from build123d import *

# Parameters (mm, degrees)
AUFSATZ_LINEAR_AUSTRAGEN1_DEPTH = 3
AUFSATZ_LINEAR_AUSTRAGEN2_DEPTH = 83.5
SKIZZE5_R                       = 1.05
SCHNITT_LINEAR_AUSTRAGEN2_DEPTH = 13


with BuildPart() as part:
    # Skizze2 → Aufsatz-Linear austragen1 (new body)
    with BuildSketch(Plane.XY):
        with BuildLine():
            ThreePointArc((18.5, 0), (13.081475452, 13.081475452), (0, 18.5))
            Line((0, 18.5), (0, 17.2))
            ThreePointArc((0, 17.2), (0.777817459, 16.877817459), (1.1, 16.1))
            ThreePointArc((1.1, 16.1), (1.099839478, 16.081208438), (1.099357959, 16.06242236))
            ThreePointArc((1.099357959, 16.06242236), (0.764416312, 15.309008406), (0, 15))
            Line((0, 15), (0, 14.3))
            ThreePointArc((0, 14.3), (0.777817459, 13.977817459), (1.1, 13.2))
            ThreePointArc((1.1, 13.2), (1.099761155, 13.177078356), (1.099044724, 13.154166667))
            ThreePointArc((1.099044724, 13.154166667), (0.761440521, 12.40614338), (0, 12.1))
            Line((0, 12.1), (0, 11.25))
            ThreePointArc((0, 11.25), (0.777817459, 10.927817459), (1.1, 10.15))
            ThreePointArc((1.1, 10.15), (1.099595894, 10.120186092), (1.098383874, 10.090394089))
            ThreePointArc((1.098383874, 10.090394089), (0.756450097, 9.35138667), (0, 9.05))
            Line((0, 9.05), (0, 8.35))
            ThreePointArc((0, 8.35), (0.777817459, 8.027817459), (1.1, 7.25))
            ThreePointArc((1.1, 7.25), (1.099207253, 7.208245771), (1.096830153, 7.166551724))
            ThreePointArc((1.096830153, 7.166551724), (0.747732204, 6.443218399), (0, 6.15))
            Line((0, 6.15), (0, 0))
            Line((0, 0), (6.15, 0))
            ThreePointArc((6.15, 0), (6.443218399, 0.747732204), (7.166551724, 1.096830153))
            ThreePointArc((7.166551724, 1.096830153), (7.997732204, 0.806781601), (8.35, 0))
            Line((8.35, 0), (9.05, 0))
            ThreePointArc((9.05, 0), (9.35138667, 0.756450097), (10.090394089, 1.098383874))
            ThreePointArc((10.090394089, 1.098383874), (10.906450097, 0.79861333), (11.25, 0))
            Line((11.25, 0), (12.1, 0))
            ThreePointArc((12.1, 0), (12.40614338, 0.761440521), (13.154166667, 1.099044724))
            ThreePointArc((13.154166667, 1.099044724), (13.961440521, 0.79385662), (14.3, 0))
            Line((14.3, 0), (15, 0))
            ThreePointArc((15, 0), (15.309008406, 0.764416312), (16.06242236, 1.099357959))
            ThreePointArc((16.06242236, 1.099357959), (16.864416312, 0.790991594), (17.2, 0))
            Line((17.2, 0), (18.5, 0))
        make_face()
        with BuildLine():
            ThreePointArc((0, -18.5), (13.081475452, -13.081475452), (18.5, 0))
            Line((18.5, 0), (17.2, 0))
            ThreePointArc((17.2, 0), (16.864416312, -0.790991594), (16.06242236, -1.099357959))
            ThreePointArc((16.06242236, -1.099357959), (15.309008406, -0.764416312), (15, 0))
            Line((15, 0), (14.3, 0))
            ThreePointArc((14.3, 0), (13.961440521, -0.79385662), (13.154166667, -1.099044724))
            ThreePointArc((13.154166667, -1.099044724), (12.40614338, -0.761440521), (12.1, 0))
            Line((12.1, 0), (11.25, 0))
            ThreePointArc((11.25, 0), (10.906450097, -0.79861333), (10.090394089, -1.098383874))
            ThreePointArc((10.090394089, -1.098383874), (9.35138667, -0.756450097), (9.05, 0))
            Line((9.05, 0), (8.35, 0))
            ThreePointArc((8.35, 0), (7.997732204, -0.806781601), (7.166551724, -1.096830153))
            ThreePointArc((7.166551724, -1.096830153), (6.443218399, -0.747732204), (6.15, 0))
            Line((6.15, 0), (0, 0))
            Line((0, 0), (0, -6.15))
            ThreePointArc((0, -6.15), (0.747732204, -6.443218399), (1.096830153, -7.166551724))
            ThreePointArc((1.096830153, -7.166551724), (1.099207253, -7.208245771), (1.1, -7.25))
            ThreePointArc((1.1, -7.25), (0.777817459, -8.027817459), (0, -8.35))
            Line((0, -8.35), (0, -9.05))
            ThreePointArc((0, -9.05), (0.756450097, -9.35138667), (1.098383874, -10.090394089))
            ThreePointArc((1.098383874, -10.090394089), (1.099595894, -10.120186092), (1.1, -10.15))
            ThreePointArc((1.1, -10.15), (0.777817459, -10.927817459), (0, -11.25))
            Line((0, -11.25), (0, -12.1))
            ThreePointArc((0, -12.1), (0.761440521, -12.40614338), (1.099044724, -13.154166667))
            ThreePointArc((1.099044724, -13.154166667), (1.099761155, -13.177078356), (1.1, -13.2))
            ThreePointArc((1.1, -13.2), (0.777817459, -13.977817459), (0, -14.3))
            Line((0, -14.3), (0, -15))
            ThreePointArc((0, -15), (0.764416312, -15.309008406), (1.099357959, -16.06242236))
            ThreePointArc((1.099357959, -16.06242236), (1.099839478, -16.081208438), (1.1, -16.1))
            ThreePointArc((1.1, -16.1), (0.777817459, -16.877817459), (0, -17.2))
            Line((0, -17.2), (0, -18.5))
        make_face()
        with BuildLine():
            Line((-17.2, 0), (-18.5, 0))
            ThreePointArc((-18.5, 0), (-13.081475452, -13.081475452), (0, -18.5))
            Line((0, -18.5), (0, -17.2))
            ThreePointArc((0, -17.2), (-0.790991594, -16.864416312), (-1.099357959, -16.06242236))
            ThreePointArc((-1.099357959, -16.06242236), (-0.764416312, -15.309008406), (0, -15))
            Line((0, -15), (0, -14.3))
            ThreePointArc((0, -14.3), (-0.79385662, -13.961440521), (-1.099044724, -13.154166667))
            ThreePointArc((-1.099044724, -13.154166667), (-0.761440521, -12.40614338), (0, -12.1))
            Line((0, -12.1), (0, -11.25))
            ThreePointArc((0, -11.25), (-0.79861333, -10.906450097), (-1.098383874, -10.090394089))
            ThreePointArc((-1.098383874, -10.090394089), (-0.756450097, -9.35138667), (0, -9.05))
            Line((0, -9.05), (0, -8.35))
            ThreePointArc((0, -8.35), (-0.806781601, -7.997732204), (-1.096830153, -7.166551724))
            ThreePointArc((-1.096830153, -7.166551724), (-0.747732204, -6.443218399), (0, -6.15))
            Line((0, -6.15), (0, 0))
            Line((0, 0), (-6.15, 0))
            ThreePointArc((-6.15, 0), (-6.443218399, -0.747732204), (-7.166551724, -1.096830153))
            ThreePointArc((-7.166551724, -1.096830153), (-7.997732204, -0.806781601), (-8.35, 0))
            Line((-8.35, 0), (-9.05, 0))
            ThreePointArc((-9.05, 0), (-9.35138667, -0.756450097), (-10.090394089, -1.098383874))
            ThreePointArc((-10.090394089, -1.098383874), (-10.906450097, -0.79861333), (-11.25, 0))
            Line((-11.25, 0), (-12.1, 0))
            ThreePointArc((-12.1, 0), (-12.40614338, -0.761440521), (-13.154166667, -1.099044724))
            ThreePointArc((-13.154166667, -1.099044724), (-13.961440521, -0.79385662), (-14.3, 0))
            Line((-14.3, 0), (-15, 0))
            ThreePointArc((-15, 0), (-15.309008406, -0.764416312), (-16.06242236, -1.099357959))
            ThreePointArc((-16.06242236, -1.099357959), (-16.864416312, -0.790991594), (-17.2, 0))
        make_face()
        with BuildLine():
            Line((0, 17.2), (0, 18.5))
            ThreePointArc((0, 18.5), (-13.081475452, 13.081475452), (-18.5, 0))
            Line((-18.5, 0), (-17.2, 0))
            ThreePointArc((-17.2, 0), (-16.864416312, 0.790991594), (-16.06242236, 1.099357959))
            ThreePointArc((-16.06242236, 1.099357959), (-15.309008406, 0.764416312), (-15, 0))
            Line((-15, 0), (-14.3, 0))
            ThreePointArc((-14.3, 0), (-13.961440521, 0.79385662), (-13.154166667, 1.099044724))
            ThreePointArc((-13.154166667, 1.099044724), (-12.40614338, 0.761440521), (-12.1, 0))
            Line((-12.1, 0), (-11.25, 0))
            ThreePointArc((-11.25, 0), (-10.906450097, 0.79861333), (-10.090394089, 1.098383874))
            ThreePointArc((-10.090394089, 1.098383874), (-9.35138667, 0.756450097), (-9.05, 0))
            Line((-9.05, 0), (-8.35, 0))
            ThreePointArc((-8.35, 0), (-7.997732204, 0.806781601), (-7.166551724, 1.096830153))
            ThreePointArc((-7.166551724, 1.096830153), (-6.443218399, 0.747732204), (-6.15, 0))
            Line((-6.15, 0), (0, 0))
            Line((0, 0), (0, 6.15))
            ThreePointArc((0, 6.15), (-0.747732204, 6.443218399), (-1.096830153, 7.166551724))
            ThreePointArc((-1.096830153, 7.166551724), (-0.806781601, 7.997732204), (0, 8.35))
            Line((0, 8.35), (0, 9.05))
            ThreePointArc((0, 9.05), (-0.756450097, 9.35138667), (-1.098383874, 10.090394089))
            ThreePointArc((-1.098383874, 10.090394089), (-0.79861333, 10.906450097), (0, 11.25))
            Line((0, 11.25), (0, 12.1))
            ThreePointArc((0, 12.1), (-0.761440521, 12.40614338), (-1.099044724, 13.154166667))
            ThreePointArc((-1.099044724, 13.154166667), (-0.79385662, 13.961440521), (0, 14.3))
            Line((0, 14.3), (0, 15))
            ThreePointArc((0, 15), (-0.764416312, 15.309008406), (-1.099357959, 16.06242236))
            ThreePointArc((-1.099357959, 16.06242236), (-0.790991594, 16.864416312), (0, 17.2))
        make_face()
    extrude(amount=AUFSATZ_LINEAR_AUSTRAGEN1_DEPTH)

    # Skizze4 → Aufsatz-Linear austragen2 (add)
    with BuildSketch(Plane.XY.offset(3)):
        Polygon((2.828427125, 6.363961031), (10.960155108, 14.495689014), (14.495689014, 10.960155108), (6.363961031, 2.828427125), align=None)
        Polygon((6.363961031, -2.828427125), (14.495689014, -10.960155108), (10.960155108, -14.495689014), (2.828427125, -6.363961031), align=None)
        Polygon((-2.828427125, -6.363961031), (-10.960155108, -14.495689014), (-14.495689014, -10.960155108), (-6.363961031, -2.828427125), align=None)
        Polygon((-6.363961031, 2.828427125), (-14.495689014, 10.960155108), (-10.960155108, 14.495689014), (-2.828427125, 6.363961031), align=None)
    extrude(amount=AUFSATZ_LINEAR_AUSTRAGEN2_DEPTH)

    # Skizze5 → Schnitt-Linear austragen2 (cut)
    with BuildSketch(Plane.XY.offset(86.5)):
        with Locations((-8.66205807, -8.66205807)):
            Circle(SKIZZE5_R)
        with Locations((-8.66205807, 8.66205807)):
            Circle(SKIZZE5_R)
        with Locations((8.66205807, 8.66205807)):
            Circle(SKIZZE5_R)
        with Locations((8.66205807, -8.66205807)):
            Circle(SKIZZE5_R)
    extrude(amount=-SCHNITT_LINEAR_AUSTRAGEN2_DEPTH, mode=Mode.SUBTRACT)


solid = part.part
Geometry: final body of the model. Coordinates: model frame, mm. A direction names the side the tool comes from. Give positions to 0.01 mm unless a question says otherwise; leave off trailing zeros. Loops run counter-clockwise (first coordinate to the right, second up) from the corner with the lowest first, then second, coordinate; pieces in that order, holes last. Notation, with made-up numbers: M 15,62 L 65,62 A8 ccw 65,69 Z; hole C 27,80 d6. An arc over 180 degrees is marked long. Put each result on its own line as item: value. Start each with the question number.
1) Pull-direction query (Y, two-part tool) for faces 5 (the flat face through (-7, -9, 86.5)), 6 (the cylindrical face through (-8.89, 7.637, 80.091)), 7 (the flat face through (6.837, 10.373, 44.166)); classes: pulls with the +Y half, pulls with the -Y half, needs draft (parallel to the pull), parting line crosses it, or undercut.
2) Cut plane C-C (x = -5). Output: boundary loops of the cut face in (y, z), then the cut area to 3 significant figures.
3) Cut plane A-A (z = 57). Output: boundary loops of the cut face in (x, y).
4) Contact query for flat-ended pins moving along their axis: pin 1 (1.5 mm diameter, centred on x = -7.5, z = 10.5, fed in from -Y); pin 2 (6 mm diameter, centred on x = -3, z = 67.5, fed in from -Y); pin 3 (8 mm diameter, centred on x = -11.5, z = 50.5, fed in from -Y). Output: stop coordinate, or through.
5) Access query for faces 1 (the flat face through (10.487, 6.951, 44.166)), 2 (the flat face through (-10.487, -6.951, 44.166)), 3 (the flat face through (-6.951, 10.487, 44.166)), 4 (the flat face through (-9, -9, 73.5)). Directions: +Z, -Z, +X, -X, +Y, -Y. A direction counts if a zero-diameter tool reaches every point of the face in a straight line with its end or side. Return the directions, or none.
6) Cut plane B-B (z = 81.5). Output: boundary loops of the cut face in (x, y).
7) Ray query, line 1 along Z through (x, y) = (-16, 5); line 2 along X through (y, z) = (-7, 81.5). Return the intervals inside material, ascending.
Verdict:
1. face 5: needs draft
1. face 6: undercut
1. face 7: pulls with the +Y half
2. outline: M -17.81,0 L 17.81,0 L 17.81,3 L 8.54,3 L 8.54,86.5 L 4.19,86.5 L 4.19,3 L -4.19,3 L -4.19,86.5 L -8.54,86.5 L -8.54,3 L -17.81,3 Z
2. area: 832 mm2
3. outline: M -14.5,-10.96 L -10.96,-14.5 L -2.83,-6.36 L -6.36,-2.83 Z; M -14.5,10.96 L -6.36,2.83 L -2.83,6.36 L -10.96,14.5 Z; M 2.83,-6.36 L 10.96,-14.5 L 14.5,-10.96 L 6.36,-2.83 Z; M 2.83,6.36 L 6.36,2.83 L 14.5,10.96 L 10.96,14.5 Z
4. pin 1: y = -11.79
4. pin 2: y = -9.54
4. pin 3: y = -14.5
5. face 1: +Z, +X
5. face 2: +Z, -X
5. face 3: +Z, +Y
5. face 4: +Z
6. outline: M -14.5,-10.96 L -10.96,-14.5 L -2.83,-6.36 L -6.36,-2.83 Z; M -14.5,10.96 L -6.36,2.83 L -2.83,6.36 L -10.96,14.5 Z; M 2.83,-6.36 L 10.96,-14.5 L 14.5,-10.96 L 6.36,-2.83 Z; M 2.83,6.36 L 6.36,2.83 L 14.5,10.96 L 10.96,14.5 Z; hole C -8.66,-8.66 d2.1; hole C -8.66,8.66 d2.1; hole C 8.66,-8.66 d2.1; hole C 8.66,8.66 d2.1
7. line 1: 0 to 3
7. line 2: -10.54 to -3.46, 3.46 to 10.54
